```python
from build123d import *

# Parameters (mm, degrees)
EXTRUDE_1_DEPTH     = 4
SKETCH_2_R          = 1.65
CUT_EXTRUDE_1_DEPTH = 2.1
SKETCH_3_R          = 3
SKETCH_3_R_2        = 4
EXTRUDE_2_DEPTH     = 5.149949226
SKETCH_4_R          = 0.95
CUT_EXTRUDE_2_DEPTH = 5
CHAMFER_1_SIZE      = 0.6
CHAMFER_1_SIZE2     = 1.039230485


with BuildPart() as part:
    # 草图1 → 凸台-拉伸1 (new body)
    with BuildSketch(Plane(origin=(0, 0, 0), x_dir=(1, 0, 0), z_dir=(0, 1, 0))):
        with BuildLine():
            Line((73.808488593, -15.628718768), (68.271134495, -19.954973934))
            ThreePointArc((68.271134495, -19.954973934), (66.16306925, -20.176540519), (65.039811544, -18.378952427))
            Line((65.039811544, -18.378952427), (65.039811544, 22.170687243))
            ThreePointArc((65.039811544, 22.170687243), (66.16306925, 23.968275336), (68.271134495, 23.74670875))
            Line((68.271134495, 23.74670875), (73.808488593, 19.420453584))
            ThreePointArc((73.808488593, 19.420453584), (75.916553838, 19.198886999), (77.039811544, 20.996475091))
            Line((77.039811544, 20.996475091), (77.039811544, 66.895867408))
            Line((77.039811544, 66.895867408), (-87.960188456, 66.895867408))
            ThreePointArc((-87.960188456, 66.895867408), (-98.566790174, 62.502469126), (-102.960188456, 51.895867408))
            Line((-102.960188456, 51.895867408), (-102.960188456, -48.104132592))
            ThreePointArc((-102.960188456, -48.104132592), (-98.566790174, -58.71073431), (-87.960188456, -63.104132592))
            Line((-87.960188456, -63.104132592), (77.039811544, -63.104132592))
            Line((77.039811544, -63.104132592), (77.039811544, -17.204740275))
            ThreePointArc((77.039811544, -17.204740275), (75.916553838, -15.407152182), (73.808488593, -15.628718768))
        make_face()
    extrude(amount=EXTRUDE_1_DEPTH)

    # 草图2 → 切除-拉伸1 (cut)
    with BuildSketch(Plane(origin=(0, 4, 0), x_dir=(1, 0, 0), z_dir=(0, 1, 0))):
        with Locations(Location((72.839811544, -21.715408726, 0), (0, 0, 270))):
            Circle(SKETCH_2_R)
        with Locations(Location((71.125155248, -58.104132592, 0), (0, 0, 270))):
            Circle(SKETCH_2_R)
        with Locations(Location((52.125155248, -58.104132592, 0), (0, 0, 270))):
            Circle(SKETCH_2_R)
        with Locations(Location((33.125155248, -58.104132592, 0), (0, 0, 270))):
            Circle(SKETCH_2_R)
        with Locations(Location((14.125155248, -58.104132592, 0), (0, 0, 270))):
            Circle(SKETCH_2_R)
        with Locations(Location((-4.874844752, -58.104132592, 0), (0, 0, 270))):
            Circle(SKETCH_2_R)
        with Locations(Location((-23.874844752, -58.104132592, 0), (0, 0, 270))):
            Circle(SKETCH_2_R)
        with Locations(Location((-42.874844752, -58.104132592, 0), (0, 0, 270))):
            Circle(SKETCH_2_R)
        with Locations(Location((-61.874844752, -58.104132592, 0), (0, 0, 270))):
            Circle(SKETCH_2_R)
        with Locations(Location((-94.324149487, -54.468093622, 0), (0, 0, 270))):
            Circle(SKETCH_2_R)
        with Locations(Location((-97.960188456, 12.810523704, 0), (0, 0, 270))):
            Circle(SKETCH_2_R)
        with Locations(Location((-97.960188456, 28.810523704, 0), (0, 0, 270))):
            Circle(SKETCH_2_R)
        with Locations(Location((-97.960188456, 44.810523704, 0), (0, 0, 270))):
            Circle(SKETCH_2_R)
        with Locations(Location((-94.324149487, 58.259828439, 0), (0, 0, 270))):
            Circle(SKETCH_2_R)
        with Locations(Location((71.125155248, 61.895867408, 0), (0, 0, 270))):
            Circle(SKETCH_2_R)
        with Locations(Location((52.125155248, 61.895867408, 0), (0, 0, 270))):
            Circle(SKETCH_2_R)
        with Locations(Location((33.125155248, 61.895867408, 0), (0, 0, 270))):
            Circle(SKETCH_2_R)
        with Locations(Location((14.125155248, 61.895867408, 0), (0, 0, 270))):
            Circle(SKETCH_2_R)
        with Locations(Location((-4.874844752, 61.895867408, 0), (0, 0, 270))):
            Circle(SKETCH_2_R)
        with Locations(Location((-23.874844752, 61.895867408, 0), (0, 0, 270))):
            Circle(SKETCH_2_R)
        with Locations(Location((-42.874844752, 61.895867408, 0), (0, 0, 270))):
            Circle(SKETCH_2_R)
        with Locations(Location((-61.874844752, 61.895867408, 0), (0, 0, 270))):
            Circle(SKETCH_2_R)
        with Locations(Location((-80.874844752, 61.895867408, 0), (0, 0, 270))):
            Circle(SKETCH_2_R)
    extrude(amount=-CUT_EXTRUDE_1_DEPTH, mode=Mode.SUBTRACT)

    # 草图3 → 凸台-拉伸2 (add)
    with BuildSketch(Plane(origin=(0, 4, 0), x_dir=(1, 0, 0), z_dir=(0, 1, 0))):
        with Locations((-89.693868923, 4.986273809)):
            Circle(SKETCH_3_R)
        with Locations((-89.693868923, -46.719829823)):
            Circle(SKETCH_3_R)
        with Locations((-64.674818885, -36.171808487)):
            Circle(SKETCH_3_R_2)
        with Locations((-64.674818885, -5.561747527)):
            Circle(SKETCH_3_R_2)
    extrude(amount=EXTRUDE_2_DEPTH)

    # 草图4 → 切除-拉伸2 (cut)
    with BuildSketch(Plane(origin=(0, 9.149949226, 0), x_dir=(1, 0, 0), z_dir=(0, 1, 0))):
        with Locations(Location((-89.693868923, -46.719829823, 0), (0, 0, 180))):
            Circle(SKETCH_4_R)
        with Locations(Location((-64.674818885, -36.171808487, 0), (0, 0, 180))):
            Circle(SKETCH_4_R)
        with Locations(Location((-64.674818885, -5.561747527, 0), (0, 0, 180))):
            Circle(SKETCH_4_R)
        with Locations(Location((-89.693868923, 4.986273809, 0), (0, 0, 180))):
            Circle(SKETCH_4_R)
    extrude(amount=-CUT_EXTRUDE_2_DEPTH, mode=Mode.SUBTRACT)

    # 倒角1
    chamfer_1_edges = [part.edges().sort_by_distance(p)[0] for p in [
        (-92.693868923, 4, -4.986273809),
        (-92.693868923, 4, 46.719829823),
        (-68.674818885, 4, 36.171808487),
        (-68.674818885, 4, 5.561747527),
    ]]
    chamfer_1_side = [part.faces().sort_by_distance(p)[0] for p in [
        (-13.877724131, 4, -2.010371092),
    ]]
    chamfer(chamfer_1_edges, length=CHAMFER_1_SIZE, length2=CHAMFER_1_SIZE2, reference=chamfer_1_side[0])


solid = part.part
```
Design review of the part built by this model. Coordinates are the model's own, in mm. A direction names the side the tool comes from. Give positions to 0.01 mm unless a question says otherwise; leave off trailing zeros. Write each loop counter-clockwise with the first axis right and the second up, starting at its lowest first coordinate (ties: lowest second). Pieces come first, ordered by that corner, then holes. Notation, with made-up numbers: (-26.5, 33.25) -> (25.5, 33.25) arc R8 ccw to (25.5, 47.25) -> close; hole circle Ø4 at (-10, 21.5). An arc over 180 degrees is marked (long way). Answer in a Markdown table with one row per item.
(1) Clearance check with flat-ended pins moving along their axes: pin 1 (2.5 mm diameter, centred on x = 70.5, z = -62.5, fed in from +Y); pin 2 (1.5 mm diameter, centred on y = 2.5, z = -2.5, fed in from +X); pin 3 (1.6 mm diameter, centred on x = -81.5, z = -61.5, fed in from +Y). State where each tip first meets the part, or that it passes through.
Results:
| item | result |
|---|---|
| pin 1 | y = 4 |
| pin 2 | x = 65.04 |
| pin 3 | y = 1.9 |
(2) Consider section A-A (y = 6.75). State the section outline as (x, z) points.
Results:
| item | result |
|---|---|
| outline | circle Ø6 at (-89.69, -4.99); circle Ø6 at (-89.69, 46.72); circle Ø8 at (-64.67, 5.56); circle Ø8 at (-64.67, 36.17); hole circle Ø1.9 at (-89.69, -4.99); hole circle Ø1.9 at (-89.69, 46.72); hole circle Ø1.9 at (-64.67, 5.56); hole circle Ø1.9 at (-64.67, 36.17) |
(3) Consider section B-B (x = 27). State the section outline as (y, z) points, then the cut area to 3 significant figures.
Results:
| item | result |
|---|---|
| outline | (0, -66.9) -> (4, -66.9) -> (4, 63.1) -> (0, 63.1) -> close |
| area | 520 mm2 |
(4) To check wall thickness, follow probe 1 along X at (y, z) = (8.5, -5); probe 2 along Z at (x, y) = (-60.5, 2.5); probe 3 along Y at (x, z) = (-27, -47.5). State the ranges of each line that lie inside material, in increasing order.
Results:
| item | result |
|---|---|
| probe 1 | -92.69 to -90.64, -88.74 to -86.69 |
| probe 2 | -66.9 to -62.81, -60.98 to 57.19, 59.02 to 63.1 |
| probe 3 | 0 to 4 |
(5) For faces 4 (the cylindrical face through (-60.98, 7.07, 37.7)), 5 (the flat face through (-90, 9.15, 48)), 6 (the flat face through (65.04, 2, -2)), list the 3-axis set-ups (+Z, -Z, +X, -X, +Y, -Y) from which the entire face can be reached by the end or side of a thin tool; tool diameter is ignored.
Results:
| item | result |
|---|---|
| face 4 | +Y |
| face 5 | +Z, -Z, +X, -X, +Y |
| face 6 | +Y, -Y |
(6) Mouldability with a two-part tool opening along X and no side actions: class faces 1 (the cylindrical face through (-92.69, 7.07, 46.59)), 2 (the flat face through (71.001, 1.972, -21.614)), 3 (the cylindrical face through (-98.45, 1.97, -62.62)) as +X half, -X half, draft (parallel to the pull), parting line (faces both ways), or undercut.
Results:
| item | result |
|---|---|
| face 1 | parting line |
| face 2 | undercut |
| face 3 | -X half |
